Model file for the job. Use its own axes, mm. A direction names the side the tool comes from. Round coordinates to 2 decimals unless told otherwise and drop trailing zeros. Order: outer loops, then holes, each group sorted by start corner. A loop starts at its lowest first (then second) coordinate and runs counter-clockwise, first axis right, second up. Notation, with made-up numbers: (-20, -18) -> (33, -18) arc R30 ccw to (33, 4) -> close; hole circle Ø7 at (-32.5, -16.75). An arc over 180 degrees is marked (long way). Put each result on its own line as item: value. Start each with the question number.
Q1. Cut at C-C, the plane z = 3.5. List the corners of the cut face in (x, y).
Q2. Flat gauge pin, fed straight in: P1, Ø4.5, axis at x = 9.5, y = 6.5, coming from the -Z side. Where does the tip first touch, or does it go through?
Q3. 3-axis set-ups, long thin cutter, end or side, ignore diameter. For faces 5 (the face through (18.936, 10.899, 2.52)), 6 (the face through (10, 6, 3)): which of +Z, -Z, +X, -X, +Y, -Y reach the whole face in a straight line?
Q4. Probe L1, parallel to X at y = 5.75, z = 2.3; L2, parallel to X at y = 4.25, z = 0.9; L3, parallel to Y at x = 11.75, z = 1.65. List the from-to ranges inside material, lowest first.
Q5. Cut at B-B, the plane y = 5.75. List the corners of the cut face in (x, z).
Q6. Cut at A-A, the plane z = 1.5. List the corners of the cut face in (x, y).
Q7. Cut at D-D, the plane x = 1. List the corners of the cut face in (y, z), and give its area (3 significant figures).
Q8. Pull direction Y, two halves, no side cores. Call faces 1 (the face through (10, 11.5, 2)), 2 (the face through (10, 0, 2)), 3 (the face through (12, 3, 0)), 4 (the face through (9.406, 3.086, 1.479)): released by +Y, released by -Y, zero draft, split by the parting line, or undercut.
Autodesk Fusion 360 part; units mm, degrees
box "BoxPrimitive1" add length 11.5 width 19.5 height 4.97 placed x (0, 1, 0) y (-1, 0, 0) z (0, 0, 1) at (19.5059, 0, 0)
sketch "Sketch3" plane through (0, 0, 0) normal (0, 0, -1) x (1, 0, 0)
  line L0 (0.0059, -11.5) -> (19.5059, -11.5)
  line L1 (19.5059, -11.5) -> (19.5059, 0)
  line L2 (19.5059, 0) -> (0.0059, 0)
  line L3 (0.0059, 0) -> (0.0059, -11.5)
  line L4 (19.5059, -11.5) -> (0.0059, 0) construction
  line L5 (19.5059, 0) -> (0.0059, -11.5) construction
  line L6 (7.8559, -3.85) -> (11.6559, -3.85) construction
  line L7 (11.6559, -3.85) -> (11.6559, -7.65) construction
  line L8 (11.6559, -7.65) -> (7.8559, -7.65) construction
  line L9 (7.8559, -7.65) -> (7.8559, -3.85) construction
  line L10 (7.8559, -3.85) -> (11.6559, -7.65) construction
  line L11 (11.6559, -3.85) -> (7.8559, -7.65) construction
  circle A0 centre (9.7559, -5.75) radius 2.687
  point P0 (9.7559, -5.75)
  point P1 (9.7559, -5.75)
  dimension "d6" = 3.8
extrude "Extrude1" cut sketch "Sketch3" against normal blind 3 contours A0
fillet "Fillet1" radius 2 4 edges at (0.0059, 11.5, 2.485) (0.0059, 0, 2.485) (19.5059, 11.5, 2.485) (19.5059, 0, 2.485)
Ans:
1. outline: (0.01, 2) arc R2 ccw to (2.01, 0) -> (17.51, 0) arc R2 ccw to (19.51, 2) -> (19.51, 9.5) arc R2 ccw to (17.51, 11.5) -> (2.01, 11.5) arc R2 ccw to (0.01, 9.5) -> close
2. P1: stops at z = 0
3. face 5: +Z, -Z, +X, +Y
3. face 6: -Z
4. L1: x = 0.01 to 7.07, 12.44 to 19.51
4. L2: x = 0.01 to 7.53, 11.99 to 19.51
4. L3: y = 0 to 3.95, 7.55 to 11.5
5. outline: (0.01, 0) -> (7.07, 0) -> (7.07, 3) -> (12.44, 3) -> (12.44, 0) -> (19.51, 0) -> (19.51, 4.97) -> (0.01, 4.97) -> close
6. outline: (0.01, 2) arc R2 ccw to (2.01, 0) -> (17.51, 0) arc R2 ccw to (19.51, 2) -> (19.51, 9.5) arc R2 ccw to (17.51, 11.5) -> (2.01, 11.5) arc R2 ccw to (0.01, 9.5) -> close; hole circle Ø5.37 at (9.76, 5.75)
7. outline: (0.27, 0) -> (11.23, 0) -> (11.23, 4.97) -> (0.27, 4.97) -> close
7. area: 54.5 mm^2
8. face 1: released by +Y
8. face 2: released by -Y
8. face 3: zero draft
8. face 4: undercut
